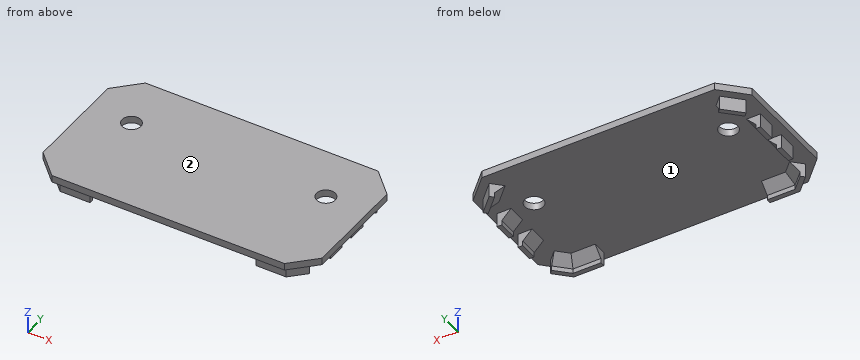
```python
from build123d import *

# Parameters (mm, degrees)
SKETCH1_W           = 120
SKETCH1_H           = 65
BOSS_EXTRUDE1_DEPTH = 3
CHAMFER1_SIZE       = 10
SKETCH2_W           = 2
SKETCH2_H           = 8
BOSS_EXTRUDE3_DEPTH = 6
CHAMFER2_SIZE       = 4
SKETCH4_R           = 4
CUT_EXTRUDE1_DEPTH  = 6


with BuildPart() as part:
    # Sketch1 → Boss-Extrude1 (new body)
    with BuildSketch(Plane.XY):
        with Locations((60, 32.5)):
            Rectangle(SKETCH1_W, SKETCH1_H)
    extrude(amount=BOSS_EXTRUDE1_DEPTH)

    # Chamfer1
    chamfer1_edges = [part.edges().sort_by_distance(p)[0] for p in [
        (0, 65, 1.5),
        (120, 65, 1.5),
        (120, 0, 1.5),
        (0, 0, 1.5),
    ]]
    chamfer(chamfer1_edges, length=CHAMFER1_SIZE)

    # Sketch2 → Boss-Extrude3 (add)
    with BuildSketch(Plane(origin=(0, 0, 0), x_dir=(-1, 0, 0), z_dir=(0, 0, -1))):
        with Locations((-115.6, 25.242640687)):
            Rectangle(SKETCH2_W, SKETCH2_H)
        with Locations((-115.6, 39.757359313)):
            Rectangle(SKETCH2_W, SKETCH2_H)
        Polygon((-109.528932188, 60.6627417), (-116.6, 53.591673888), (-115.185786438, 52.177460326), (-108.114718626, 59.248528137), align=None)
        Polygon((-11.885281374, 59.248528137), (-10.471067812, 60.6627417), (-3.4, 53.591673888), (-4.814213562, 52.177460326), align=None)
        with Locations((-4.4, 25.242640687)):
            Rectangle(SKETCH2_W, SKETCH2_H)
        with Locations((-4.4, 39.757359313)):
            Rectangle(SKETCH2_W, SKETCH2_H)
        Polygon((-114.834314575, 9.642640687), (-113.420101013, 11.056854249), (-107.763246763, 5.4), (-95.763246763, 5.4), (-95.763246763, 3.4), (-108.591673888, 3.4), align=None)
        Polygon((-11.408326112, 3.4), (-5.165685425, 9.642640687), (-6.579898987, 11.056854249), (-12.236753237, 5.4), (-24.236753237, 5.4), (-24.236753237, 3.4), align=None)
    extrude(amount=BOSS_EXTRUDE3_DEPTH)

    # Chamfer2
    chamfer2_edges = [part.edges().sort_by_distance(p)[0] for p in [
        (8.349747468, 55.712994231, 0),
        (5.4, 25.242640687, 0),
        (5.4, 39.757359313, 0),
        (114.6, 39.757359313, 0),
        (114.6, 25.242640687, 0),
        (101.763246763, 5.4, 0),
        (110.591673888, 8.228427125, 0),
        (111.650252532, 55.712994231, 0),
        (9.408326112, 8.228427125, 0),
        (18.236753237, 5.4, 0),
    ]]
    chamfer(chamfer2_edges, length=CHAMFER2_SIZE)

    # Sketch4 → Cut-Extrude1 (cut)
    with BuildSketch(Plane(origin=(0, 0, 0), x_dir=(-1, 0, 0), z_dir=(0, 0, -1))):
        with Locations((-18.2, 42)):
            Circle(SKETCH4_R)
        with Locations((-101.8, 42)):
            Circle(SKETCH4_R)
    extrude(amount=-CUT_EXTRUDE1_DEPTH, mode=Mode.SUBTRACT)


solid = part.part
```
Design review of the part built by this model. Coordinates are the model's own, in mm. Face numbers are marked on the shaded views. Give positions to 0.01 mm unless a question says otherwise; leave off trailing zeros. Write each loop counter-clockwise with the first axis right and the second up, starting at its lowest first coordinate (ties: lowest second). Pieces come first, ordered by that corner, then holes. Notation, with made-up numbers: (13.25, 43.5) -> (20.25, 43.5) arc R14 cw to (20.25, 51.5) -> close; hole circle Ø2 at (89.5, -24.75). An arc over 180 degrees is marked (long way). Answer in a Markdown table with one row per item.
(1) Consider section A-A (y = 42). State the section outline as (x, z) points, then the cut area to 3 significant figures.
Results:
| item | result |
|---|---|
| outline | (0, 0) -> (3.4, 0) -> (3.4, -6) -> (5.4, -6) -> (5.4, -4) -> (9.4, 0) -> (14.2, 0) -> (14.2, 3) -> (0, 3) -> close; (22.2, 0) -> (97.8, 0) -> (97.8, 3) -> (22.2, 3) -> close; (105.8, 0) -> (110.6, 0) -> (114.6, -4) -> (114.6, -6) -> (116.6, -6) -> (116.6, 0) -> (120, 0) -> (120, 3) -> (105.8, 3) -> close |
| area | 352 mm2 |
(2) Consider section D-D (x = 67). State the section outline as (y, z) points.
Results:
| item | result |
|---|---|
| outline | (0, 0) -> (65, 0) -> (65, 3) -> (0, 3) -> close |
(3) Clearance check with flat-ended pins moving along their axes: pin 1 (3 mm diameter, centred on x = 6, z = -4, fed in from +Y); pin 2 (7 mm diameter, centred on x = 101.8, y = 42, fed in from -Z); pin 3 (1.6 mm diameter, centred on y = 40, z = -4.5, fed in from -X); pin 4 (3 mm diameter, centred on x = 7.5, z = -3, fed in from +Y). State where each tip first meets the part, or that it passes through.
Results:
| item | result |
|---|---|
| pin 1 | y = 57.69 |
| pin 2 | through |
| pin 3 | x = 3.4 |
| pin 4 | y = 59.19 |
(4) Mouldability with a two-part tool opening along X and no side actions: class the marked faces 1 and 2 as +X half, -X half, draft (parallel to the pull), parting line (faces both ways), or undercut.
Results:
| item | result |
|---|---|
| face 1 | undercut |
| face 2 | draft |
(5) Consider section C-C (y = 27). State the section outline as (x, z) points, then the cut area to 3 significant figures.
Results:
| item | result |
|---|---|
| outline | (0, 0) -> (3.4, 0) -> (3.4, -6) -> (5.4, -6) -> (5.4, -4) -> (9.4, 0) -> (110.6, 0) -> (114.6, -4) -> (114.6, -6) -> (116.6, -6) -> (116.6, 0) -> (120, 0) -> (120, 3) -> (0, 3) -> close |
| area | 400 mm2 |
(6) Consider section B-B (x = 18.2). State the section outline as (y, z) points.
Results:
| item | result |
|---|---|
| outline | (0, 0) -> (3.4, 0) -> (3.4, -6) -> (5.4, -6) -> (5.4, -4) -> (9.4, 0) -> (38, 0) -> (38, 3) -> (0, 3) -> close; (46, 0) -> (65, 0) -> (65, 3) -> (46, 3) -> close |
(7) To check wall thickness, follow probe 1 along Y at (x, z) = (18.2, 0.9); probe 2 along X at (y, z) = (39, -5.5); probe 3 along Z at (x, y) = (66.5, 22). State the ranges of each line that lie inside material, in increasing order.
Results:
| item | result |
|---|---|
| probe 1 | 0 to 38, 46 to 65 |
| probe 2 | 3.4 to 5.4, 114.6 to 116.6 |
| probe 3 | 0 to 3 |
